Work out the finished part from the listing and answer in its coordinate system (mm). Coordinates: 2 decimals unless noted, no trailing zeros. Order: outer loops, then holes, each group sorted by start corner. A loop starts at its lowest first (then second) coordinate and runs counter-clockwise, first axis right, second up. Notation, with made-up numbers: M 59.5,84.25 L 96.5,84.25 A22 ccw 96.5,116.25 Z; hole C 86,56 d4. An arc over 180 degrees is marked long. Answer in a Markdown table with one row per item. Add a question column.
Item 1: The part is cut by section C-C (x = 114.3). Write down the section's boundary in (y, z), then the cut area to 3 significant figures.
Item 2: The part is cut by section B-B (y = -2.25). Write down the section's boundary in (x, z), then the cut area to 3 significant figures.
Item 3: The part is cut by section A-A (x = 44.45). Write down the section's boundary in (y, z), then the cut area to 3 significant figures.
Item 4: The part is cut by section D-D (z = 16). Write down the section's boundary in (x, y), then the cut area to 3 significant figures.
Item 5: Flat-ended cylindrical pins translate along their axes: pin 1 Ø1.5 at (x, y) = (129, -2) entering from +Z; pin 2 Ø23 at (x, z) = (44.45, 63.62) entering from -Y. Find the tip coordinate at first contact, or state that the pin passes through.
Item 6: Consider line 1 (X direction, y = -3.15, z = 66); line 2 (X direction, y = -3.8, z = 61); line 3 (Z direction, x = 114.3, y = -2.7). Determine where each line is inside the solid, lowest interval first. Write a range as from..to.
from build123d import *

# Parameters (mm, degrees)
F1_DEPTH = 4.7625
F2_R     = 19.05
F2_R_2   = 6.35
F3_DEPTH = 4.7635


with BuildPart() as f1:
    # F0 (on Front) → F1 (new body)
    with BuildSketch(Plane.XZ):
        with BuildLine():
            Line((0, 111.24605), (0, -3.05395))
            Line((0, -3.05395), (165.1, -3.05395))
            ThreePointArc((165.1, -3.05395), (140.608839, 63.168609), (88.9, 111.24605))
            Line((88.9, 111.24605), (0, 111.24605))
        make_face()
    extrude(amount=F1_DEPTH)

    # F2 (on face) → F3 (cut, through all)
    with BuildSketch(Plane.XZ.offset(4.7625)):
        with Locations((44.45, 63.62105)):
            Circle(F2_R)
        with Locations((114.3, 63.62105)):
            Circle(F2_R_2)
    extrude(amount=-F3_DEPTH, mode=Mode.SUBTRACT)


solid = f1.part
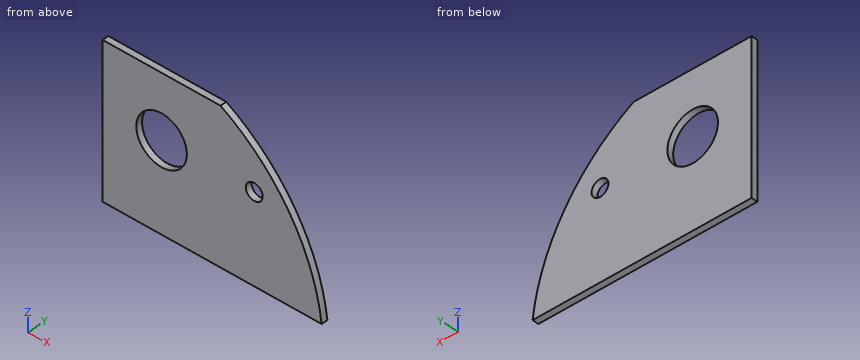
Reply:
| question | item | result |
|---|---|---|
| 1 | outline | M -4.76,-3.05 L 0,-3.05 L 0,57.27 L -4.76,57.27 Z; M -4.76,69.97 L 0,69.97 L 0,93.2 L -4.76,93.2 Z |
| 1 | area | 398 mm2 |
| 2 | outline | M 0,-3.05 L 165.1,-3.05 A152.4 ccw 88.9,111.25 L 0,111.25 Z; hole C 44.45,63.62 d38.1; hole C 114.3,63.62 d12.7 |
| 2 | area | 14,800 mm2 |
| 3 | outline | M -4.76,-3.05 L 0,-3.05 L 0,44.57 L -4.76,44.57 Z; M -4.76,82.67 L 0,82.67 L 0,111.25 L -4.76,111.25 Z |
| 3 | area | 363 mm2 |
| 4 | outline | M 0,-4.76 L 161.55,-4.76 L 161.55,0 L 0,0 Z |
| 4 | area | 769 mm2 |
| 5 | pin 1 | stops at z = 79.27 |
| 5 | pin 2 | passes through |
| 6 | line 1 | x = 0..25.55, 63.35..108.41, 120.19..138.67 |
| 6 | line 2 | x = 0..25.58, 63.32..108.52, 120.08..142.03 |
| 6 | line 3 | z = -3.05..57.27, 69.97..93.2 |
